Check sheet for the modelled part. Datum: model origin and axes. Units: mm. Face numbers are marked on the shaded views. A direction names the side the tool comes from. Round coordinates to 2 decimals unless told otherwise and drop trailing zeros. Order: outer loops, then holes, each group sorted by start corner. A loop starts at its lowest first (then second) coordinate and runs counter-clockwise, first axis right, second up. Notation, with made-up numbers: (68.5, 20) -> (72.5, 20) arc R14 ccw to (72.5, 46) -> close; hole circle Ø6 at (17, 65). An arc over 180 degrees is marked (long way). Use CSV: the item, a comma, the result in double quotes.
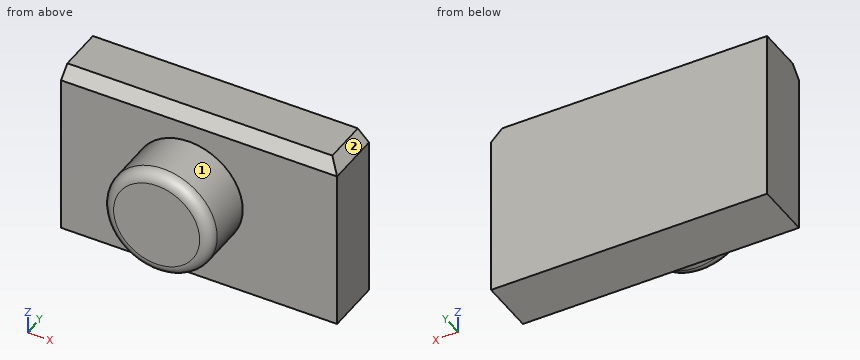
```python
from build123d import *

# Parameters (mm, degrees)
F0_W     = 125.596717
F0_H     = 78.660075
F1_DEPTH = 25.4
F2_SIZE  = 5.08
F3_R     = 24.65401
F4_DEPTH = 25.4
F5_R     = 5.08


with BuildPart() as f1:
    # F0 (on Front) → F1 (new body)
    with BuildSketch(Plane.XZ):
        with Locations((4.805998, -1.282626)):
            Rectangle(F0_W, F0_H)
    extrude(amount=F1_DEPTH)

    # F2
    f2_edges = [f1.edges().sort_by_distance(p)[0] for p in [
        (67.604356, -12.7, 38.047411),
        (4.805997, -25.4, 38.047411),
    ]]
    chamfer(f2_edges, length=F2_SIZE)

    # F3 (on face) → F4 (join)
    with BuildSketch(Plane.XZ.offset(25.4)):
        Circle(F3_R)
    extrude(amount=F4_DEPTH)

    # F5
    f5_edges = [f1.edges().sort_by_distance(p)[0] for p in [
        (-24.65401, -50.8, 0),
    ]]
    fillet(f5_edges, radius=F5_R)


solid = f1.part
```
Q1. Access from +Z, -Z, +X, -X, +Y, -Y to the whole of each face (thin tool, end or side, straight path). Record for the marked faces 1 and 2.
Result sheet:
face 1,"-Y"
face 2,"+Z, +X, +Y, -Y"
Q2. Sectioned sample at C-C, the plane y = -30. Enter the section's corners in (x, z), then the cut area to 3 significant figures.
Result sheet:
outline,"circle Ø49.31 at (0, 0)"
area,"1,910 mm^2"
Q3. Sectioned sample at A-A, the plane x = 0. Enter the section's corners in (y, z), then the cut area to 3 significant figures.
Result sheet:
outline,"(-50.8, -19.57) arc R5.08 ccw to (-45.72, -24.65) -> (-25.4, -24.65) -> (-25.4, -40.61) -> (0, -40.61) -> (0, 38.05) -> (-20.32, 38.05) -> (-25.4, 32.97) -> (-25.4, 24.65) -> (-45.72, 24.65) arc R5.08 ccw to (-50.8, 19.57) -> close"
area,"3,230 mm^2"
Q4. Sectioned sample at D-D, the plane x = -27. Enter the section's corners in (y, z).
Result sheet:
outline,"(-25.4, -40.61) -> (0, -40.61) -> (0, 38.05) -> (-20.32, 38.05) -> (-25.4, 32.97) -> close"
Q5. Scan lines: L1, parallel to X at y = -46, z = 1; L2, parallel to Y at x = 47, z = 13; L3, parallel to X at y = -31.5, z = 4.5. Record each from-to range of solid material in increasing order.
Result sheet:
L1,"x = -24.63 to 24.63"
L2,"y = -25.4 to 0"
L3,"x = -24.24 to 24.24"
Q6. Go/stop test with flat-tipped pins: pin 1 (3 mm diameter, centred on x = -41.5, z = 28.5, fed in from -Y); pin 2 (12 mm diameter, centred on x = -21, y = -37, fed in from +Z). Record where each tip stops, or that it passes through.
Result sheet:
pin 1,"stops at y = -25.4"
pin 2,"stops at z = 19.57"
Q7. Sectioned sample at B-B, the plane z = 0. Enter the section's corners in (x, y).
Result sheet:
outline,"(-57.99, -25.4) -> (-24.65, -25.4) -> (-24.65, -45.72) arc R5.08 ccw to (-19.57, -50.8) -> (19.57, -50.8) arc R5.08 ccw to (24.65, -45.72) -> (24.65, -25.4) -> (67.6, -25.4) -> (67.6, 0) -> (-57.99, 0) -> close"
